Check sheet for the modelled part. Datum: model origin and axes. Units: mm. A direction names the side the tool comes from. Round coordinates to 2 decimals unless told otherwise and drop trailing zeros. Loops run counter-clockwise (first coordinate to the right, second up) from the corner with the lowest first, then second, coordinate; pieces in that order, holes last. Notation, with made-up numbers: (-37, 44.5) -> (6, 44.5) arc R21 cw to (6, 55.5) -> close; hole circle Ø5 at (-28.5, 73). An arc over 180 degrees is marked (long way). One line per item, written item: value. Start each with the question number.
1. Set-up check for faces 1 (the face through (0, 0, -68.26)), 2 (the face through (0, 0, -68.895)), 3 (the face through (-5, -12, -94.295)): record each of +Z, -Z, +X, -X, +Y, -Y from which the full face is reachable in a straight line by a thin tool's end or side.
2. Cross-section at B-B on z = -57.5. Record the cut outline in (x, y).
3. Cross-section at A-A on z = 25. Record the cut outline in (x, y).
4. Go/stop test with flat-tipped pins: pin 1 (3 mm diameter, centred on y = -35, z = 19, fed in from +X); pin 2 (5 mm diameter, centred on y = 28, z = -24.5, fed in from +X); pin 3 (4 mm diameter, centred on x = -12.5, z = -67.5, fed in from +Y). Record where each tip stops, or that it passes through.
5. Material ranges on L1, parallel to X at y = 0, z = -78 (3 decimals); L2, parallel to Y at x = 0, z = -78.75 (3 decimals); L3, parallel to X at y = 0, z = -78.5 (3 decimals), recorded low to high.
6. Release check for a two-part mould opening along X. For faces 4 (the face through (33, -20, 77.155)), 5 (the face through (1.74, -13.22, -80.98)) record: +X half, -X half, draft (parallel to the pull), parting line (faces both ways), or undercut.
from build123d import *

# Parameters (mm, degrees)
F0_W = 0.635
F0_H = 0.9395605023


with BuildPart() as f1:
    # F0 (on Front) → F1 (revolve)
    with BuildSketch(Plane.XZ):
        Polygon((-19.05, -94.2954702053), (-19.1543956114, -93.355909703), (-25.5043956114, -93.355909703), (-25.4, -94.2954702053), align=None)
        with Locations((-13.0175, -93.8256899541)):
            Rectangle(F0_W, F0_H)
        Polygon((0, -68.8954702053), (0, -68.2604702053), (-13.335, -68.2604702053), (-13.335, -93.355909703), (-12.7, -93.355909703), (-12.7, -68.8954702053), align=None)
        Polygon((-13.335, -93.355909703), (-19.1543956114, -93.355909703), (-19.05, -94.2954702053), (-13.335, -94.2954702053), align=None)
        Polygon((-19.1543956114, -93.355909703), (-38.1, 77.1545297947), (-44.45, 77.1545297947), (-25.5043956114, -93.355909703), align=None)
    revolve(axis=Axis((0, 0, 4.1295297947), (0, 0, 1)))


solid = f1.part
Taken from the geometry:
1. face 1: +Z
1. face 2: -Z
1. face 3: -Z, +X, -X, +Y, -Y
2. outline: circle Ø58.98 at (0, 0); hole circle Ø46.28 at (0, 0)
3. outline: circle Ø77.31 at (0, 0); hole circle Ø64.61 at (0, 0)
4. pin 1: stops at x = 17.93
4. pin 2: stops at x = 21.22
4. pin 3: stops at y = 26.4
5. L1: x = -27.211 to -20.861, -13.335 to -12.7, 12.7 to 13.335, 20.861 to 27.211
5. L2: y = -27.127 to -20.777, -13.335 to -12.7, 12.7 to 13.335, 20.777 to 27.127
5. L3: x = -27.155 to -20.805, -13.335 to -12.7, 12.7 to 13.335, 20.805 to 27.155
6. face 4: draft
6. face 5: undercut
